Can you work these out from the model? Positions are in its coordinate system, mm. Round coordinates to 2 decimals unless told otherwise and drop trailing zeros. Write each loop counter-clockwise with the first axis right and the second up, starting at its lowest first coordinate (ties: lowest second). Pieces come first, ordered by that corner, then holes.
Q1. If we section it at B-B (x = 0): Please give me the cut outline in (y, z) (3 decimals), plus the area to 3 significant figures.
Q2. I'm going to push flat-ended pins straight in: pin 1 Ø4 at (x, y) = (24, 1.5) entering from -Z; pin 2 Ø3 at (x, y) = (27.5, -0.5) entering from -Z; pin 3 Ø4 at (x, y) = (-28, -2) entering from +Z. Where does each tip first touch, or does it pass through?
Q3. Please list where these lines run through material, in increasing order: line 1 along Y through (x, z) = (65, 0); line 2 along X through (y, z) = (1.5, 11.5); line 3 along X through (y, z) = (0.25, -4.5).
Q4. If we section it at A-A (z = 0): Please give me the cut outline in (x, y).
Q5. If we section it at D-D (x = -17): Please give me the cut outline in (y, z) (3 decimals), plus the area to 3 significant figures.
Q6. If we section it at C-C (z = 21.5): Please give me the cut outline in (x, y), plus the area to 3 significant figures.
from build123d import *

# Parameters (mm, degrees)
SKETCH1_R               = 12.7
SKETCH1_R_2             = 3.3528
BOSS_EXTRUDE1_DEPTH     = 3.81
SKETCH2_R               = 5.207
BOSS_EXTRUDE2_DEPTH     = 3.81
CUT_EXTRUDE1_REACH      = 85.81
CUT_EXTRUDE1_END_RADIUS = 5.207
SKETCH3_R               = 2.794
BOSS_EXTRUDE3_DEPTH     = 3.81
FILLET1_R               = 2.54


with BuildPart() as part:
    # Sketch1 → Boss-Extrude1 (new, symmetric)
    with BuildSketch(Plane(origin=(0, 0, 0), x_dir=(1, 0, 0), z_dir=(0, 1, 0))):
        with Locations(Location((0, 0, 0), (0, 0, 90))):
            Circle(SKETCH1_R)
        with Locations(Location((0, 0, 0), (0, 0, 90))):
            Circle(SKETCH1_R_2, mode=Mode.SUBTRACT)
    extrude(amount=BOSS_EXTRUDE1_DEPTH, both=True)

    # Sketch2 → Boss-Extrude2 (add, symmetric)
    with BuildSketch(Plane(origin=(0, 0, 0), x_dir=(1, 0, 0), z_dir=(0, 1, 0))):
        with BuildLine():
            Line((12.296722124, 3.175), (42.275578844, 3.175))
            ThreePointArc((42.275578844, 3.175), (69.85, 0), (42.275578844, -3.175))
            Line((42.275578844, -3.175), (12.296722124, -3.175))
            ThreePointArc((12.296722124, -3.175), (12.7, 0), (12.296722124, 3.175))
        make_face()
        with Locations(Location((55.88, 0, 0), (0, 0, 90))):
            Circle(SKETCH2_R, mode=Mode.SUBTRACT)
    boss_extrude2 = extrude(amount=BOSS_EXTRUDE2_DEPTH, both=True)

    # Cut-Extrude1: up to this cylinder (the profile starts outside it)
    cut_extrude1_end = Plane(origin=(55.88, 0, 0), z_dir=(0, -1, 0)) * Cylinder(CUT_EXTRUDE1_END_RADIUS, 183.034, mode=Mode.PRIVATE)
    # Sketch3 → Cut-Extrude1 (cut, up to the surface)
    with BuildSketch(Plane(origin=(69.85, 0, 0), x_dir=(0, 0, -1), z_dir=(1, 0, 0)), mode=Mode.PRIVATE) as cut_extrude1_sk1:
        Circle(SKETCH3_R)
    cut_extrude1_tool1 = extrude(cut_extrude1_sk1.sketch, amount=-CUT_EXTRUDE1_REACH, mode=Mode.PRIVATE) - cut_extrude1_end
    cut_extrude1 = cut_extrude1_tool1.solids().sort_by_distance((69.85, 0, 0))[0]
    add(cut_extrude1, mode=Mode.SUBTRACT)

    # Mirror1: Boss-Extrude2, Cut-Extrude1 across plane
    add(boss_extrude2.mirror(Plane(origin=(0, 0, 0), x_dir=(0, 0, 1), z_dir=(1, 0, 0))))
    add(cut_extrude1.mirror(Plane(origin=(0, 0, 0), x_dir=(0, 0, 1), z_dir=(1, 0, 0))), mode=Mode.SUBTRACT)

    # Sketch4 → Boss-Extrude3 (add, symmetric)
    with BuildSketch(Plane(origin=(0, 0, 0), x_dir=(1, 0, 0), z_dir=(0, 1, 0))):
        with BuildLine():
            ThreePointArc((-51.048948864, -13.10808319), (-54.178749787, -13.866024943), (-57.398948864, -13.887177336))
            ThreePointArc((-57.398948864, -13.887177336), (0, -59.055), (57.398948864, -13.887177336))
            ThreePointArc((57.398948864, -13.887177336), (54.178749787, -13.866024943), (51.048948864, -13.10808319))
            ThreePointArc((51.048948864, -13.10808319), (0, -52.705), (-51.048948864, -13.10808319))
        make_face()
        with BuildLine():
            ThreePointArc((57.398948864, 13.887177336), (0, 59.055), (-57.398948864, 13.887177336))
            ThreePointArc((-57.398948864, 13.887177336), (-54.178749787, 13.866024943), (-51.048948864, 13.10808319))
            ThreePointArc((-51.048948864, 13.10808319), (0, 52.705), (51.048948864, 13.10808319))
            ThreePointArc((51.048948864, 13.10808319), (54.178749787, 13.866024943), (57.398948864, 13.887177336))
        make_face()
    extrude(amount=BOSS_EXTRUDE3_DEPTH, both=True)

    # Fillet1
    fillet1_edges = [part.edges().sort_by_distance(p)[0] for p in [
        (12.296722124, 0, -3.175),
        (12.296722124, 0, 3.175),
        (42.275578844, 0, 3.175),
        (42.275578844, 0, -3.175),
        (-12.296722124, 0, 3.175),
        (-12.296722124, 0, -3.175),
        (-42.275578844, 0, -3.175),
        (-42.275578844, 0, 3.175),
        (-51.048948864, 0, 13.10808319),
        (-57.398948864, 0, 13.887177336),
        (57.398948864, 0, 13.887177336),
        (51.048948864, 0, 13.10808319),
        (51.048948864, 0, -13.10808319),
        (57.398948864, 0, -13.887177336),
        (-57.398948864, 0, -13.887177336),
        (-51.048948864, 0, -13.10808319),
    ]]
    fillet(fillet1_edges, radius=FILLET1_R)


solid = part.part
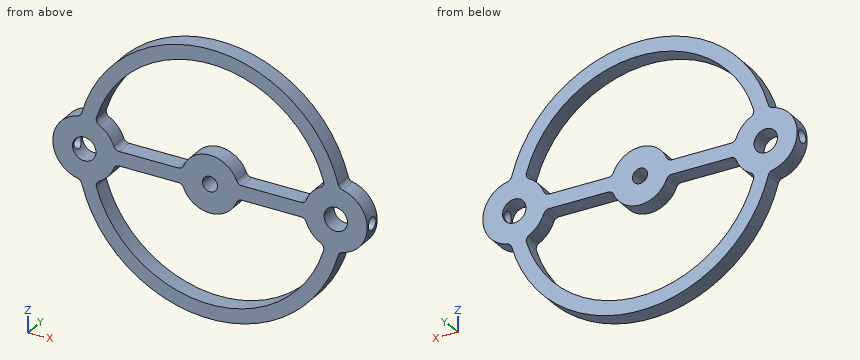
A:
1. outline: (-3.81, -59.055) - (3.81, -59.055) - (3.81, -52.705) - (-3.81, -52.705) - close; (-3.81, -12.7) - (3.81, -12.7) - (3.81, -3.353) - (-3.81, -3.353) - close; (-3.81, 3.353) - (3.81, 3.353) - (3.81, 12.7) - (-3.81, 12.7) - close; (-3.81, 52.705) - (3.81, 52.705) - (3.81, 59.055) - (-3.81, 59.055) - close
1. area: 239 mm2
2. pin 1: stops at z = -54.8
2. pin 2: stops at z = -53.02
2. pin 3: stops at z = 53.02
3. line 1: y = -3.81 to -2.79, 2.79 to 3.81
3. line 2: x = -63.81 to -47.95, -5.39 to 5.39, 47.95 to 63.81
3. line 3: x = -69.11 to -58.5, -53.26 to -42.62, -11.9 to 11.9, 42.62 to 53.26, 58.5 to 69.11
4. outline: (-69.85, -3.81) - (-61.09, -3.81) - (-61.09, -2.79) - (-69.85, -2.79) - close; (-69.85, 2.79) - (-61.09, 2.79) - (-61.09, 3.81) - (-69.85, 3.81) - close; (-50.67, -3.81) - (-3.35, -3.81) - (-3.35, 3.81) - (-50.67, 3.81) - close; (3.35, -3.81) - (50.67, -3.81) - (50.67, 3.81) - (3.35, 3.81) - close; (61.09, -3.81) - (69.85, -3.81) - (69.85, -2.79) - (61.09, -2.79) - close; (61.09, 2.79) - (69.85, 2.79) - (69.85, 3.81) - (61.09, 3.81) - close
5. outline: (-3.81, -56.555) - (3.81, -56.555) - (3.81, -49.888) - (-3.81, -49.888) - close; (-3.81, -3.175) - (3.81, -3.175) - (3.81, 3.175) - (-3.81, 3.175) - close; (-3.81, 49.888) - (3.81, 49.888) - (3.81, 56.555) - (-3.81, 56.555) - close
5. area: 150 mm2
6. outline: (-55, -3.81) - (-48.12, -3.81) - (-48.12, 3.81) - (-55, 3.81) - close; (48.12, -3.81) - (55, -3.81) - (55, 3.81) - (48.12, 3.81) - close
6. area: 105 mm2
